```python
from build123d import *
from build123d import SkipClean  # not in build123d's __all__

# Parameters (mm, degrees)
F1_DEPTH = 10
F2_R     = 15
F3_DEPTH = 32
F4_DEPTH = 25
F5_DEPTH = 20


with BuildPart() as f1:
    # F0 (on Top) → F1 (new body)
    with BuildSketch(Plane.XY):
        with BuildLine():
            Line((-19.7133726581, 60.8366520235), (-69.7133726581, 60.8366520235))
            ThreePointArc((-69.7133726581, 60.8366520235), (-63.0146428473, 35.8366520235), (-69.7133726581, 10.8366520235))
            Line((-69.7133726581, 10.8366520235), (-19.7133726581, 10.8366520235))
            Line((-19.7133726581, 10.8366520235), (-19.7133726581, 60.8366520235))
        make_face()
    extrude(amount=F1_DEPTH)

    # F2 (on face) → F3 (join)
    with BuildSketch(Plane.XY.offset(10)):
        with Locations((-38.7318296711, 37.7283993232)):
            Circle(F2_R)
        with BuildLine():
            ThreePointArc((-35.6207755692, 50.8650405369), (-28.1429385494, 46.1024894119), (-25.2318296711, 37.7283993232))
            ThreePointArc((-25.2318296711, 37.7283993232), (-28.1429385494, 29.3543092346), (-35.6207755692, 24.5917581096))
            ThreePointArc((-35.6207755692, 24.5917581096), (-38.7318296711, 24.2283993232), (-41.8428837729, 24.5917581096))
            ThreePointArc((-41.8428837729, 24.5917581096), (-52.2318296711, 37.7283993232), (-41.8428837729, 50.8650405369))
            ThreePointArc((-41.8428837729, 50.8650405369), (-38.7318296711, 51.2283993232), (-35.6207755692, 50.8650405369))
        make_face(mode=Mode.SUBTRACT)
    extrude(amount=F3_DEPTH)

    # F2 (on face) → F4 (cut)
    with BuildSketch(Plane.XY.offset(10)):
        with BuildLine():
            Line((-41.8428837729, 24.5917581096), (-41.8428837729, 50.8650405369))
            ThreePointArc((-41.8428837729, 50.8650405369), (-52.2318296711, 37.7283993232), (-41.8428837729, 24.5917581096))
        make_face()
        with BuildLine():
            ThreePointArc((-35.6207755692, 24.5917581096), (-28.1429385494, 29.3543092346), (-25.2318296711, 37.7283993232))
            ThreePointArc((-25.2318296711, 37.7283993232), (-28.1429385494, 46.1024894119), (-35.6207755692, 50.8650405369))
            Line((-35.6207755692, 50.8650405369), (-35.6207755692, 24.5917581096))
        make_face()
    with SkipClean():  # cleaning this boolean's faces spoils the solid; the shape is the same uncleaned
        extrude(amount=-F4_DEPTH, mode=Mode.SUBTRACT)

    # F5 (add): a face of the model
    f5_faces = [f1.faces().sort_by_distance(p)[0] for p in [
        (-38.7318296711, 37.7283993232, 10),
    ]]
    with SkipClean():  # cleaning this boolean's faces spoils the solid; the shape is the same uncleaned
        extrude(f5_faces, amount=F5_DEPTH)


solid = f1.part
```
The listing builds one solid part. Answer for the finished solid, in the listing's coordinates (mm). A direction names the side the tool comes from. Round coordinates to 2 decimals unless told otherwise and drop trailing zeros. Write each loop counter-clockwise with the first axis right and the second up, starting at its lowest first coordinate (ties: lowest second). Pieces come first, ordered by that corner, then holes. Notation, with made-up numbers: (-7, 77) -> (51, 77) arc R21 cw to (51, 116) -> close; hole circle Ø8 at (62, 13). An arc over 180 degrees is marked (long way). Use CSV: the item, a comma, the result in double quotes. Start each with the question number.
(1) Section A-A on z = 6 is taken. Give the vertices of the cut face in (x, y), then the cut area to 3 significant figures.
(2) Section D-D on x = -45 is taken. Give the vertices of the cut face in (y, z).
(3) Section B-B on y = 37 is taken. Give the vertices of the cut face in (x, z), then the cut area to 3 significant figures.
(4) The mould has two halves that part along Y. Classify faces 3 (the face through (-44, 60.837, 5)), 4 (the face through (-19.713, 35, 5)), 5 (the face through (-63.016, 36.203, 4.93)), 6 (the face through (-35.621, 38, 15)): released by +Y, released by -Y, zero draft, split by the parting line, or undercut.
(5) Consider L1, parallel to X at y = 37.5, z = 32.5; L2, parallel to X at y = 35.5, z = 24.5; L3, parallel to X at y = 25.5, z = 11.5. Determine where each line is inside the solid, lowest interval first. Write a range as from..to.
(6) Each of these flat-tipped pins is pushed along its axis until it touches: pin 1 (10 mm diameter, centred on x = -32.5, z = 18.5, fed in from +Y); pin 2 (6 mm diameter, centred on y = 46, z = 21, fed in from -X) (3 decimals); pin 3 (3 mm diameter, centred on x = -40, y = 37, fed in from +Z); pin 4 (5 mm diameter, centred on x = -47.5, y = 37.5, fed in from -Z). Where does it stop, or does it pass through?
(7) Section C-C on z = 32.5 is taken. Give the vertices of the cut face in (x, y).
(8) Which of the six approach directions +Z, -Z, +X, -X, +Y, -Y give full straight-line access (tool end or side, diameter ignored) to faces 1 (the face through (-45, 10.837, 5)), 2 (the face through (-39, 38, 30))?
A:
1,outline,"(-69.71, 10.84) -> (-19.71, 10.84) -> (-19.71, 60.84) -> (-69.71, 60.84) arc R50 cw to start; hole (-41.84, 24.59) -> (-41.84, 50.87) arc R13.5 ccw to start; hole (-35.62, 24.59) arc R13.5 ccw to (-35.62, 50.87) -> close"
1,area,"1,870 mm²"
2,outline,"(10.84, 0) -> (25.77, 0) -> (25.77, 42) -> (24.1, 42) -> (24.1, 10) -> (10.84, 10) -> close; (49.68, 0) -> (60.84, 0) -> (60.84, 10) -> (51.36, 10) -> (51.36, 42) -> (49.68, 42) -> close"
3,outline,"(-63.03, 0) -> (-52.21, 0) -> (-52.21, 42) -> (-53.71, 42) -> (-53.71, 10) -> (-63.03, 10) -> close; (-41.84, 0) -> (-35.62, 0) -> (-35.62, 30) -> (-41.84, 30) -> close; (-25.25, 0) -> (-19.71, 0) -> (-19.71, 10) -> (-23.75, 10) -> (-23.75, 42) -> (-25.25, 42) -> close"
3,area,"446 mm²"
4,face 3,"released by +Y"
4,face 4,"zero draft"
4,face 5,"undercut"
4,face 6,"undercut"
5,L1,"x = -53.73..-52.23, -25.23..-23.73"
5,L2,"x = -53.57..-52.05, -41.84..-35.62, -25.42..-23.9"
5,L3,"x = -47.42..-44.45, -41.84..-35.62, -33.01..-30.04"
6,pin 1,"stops at y = 52.68"
6,pin 2,"stops at x = -52.775"
6,pin 3,"stops at z = 30"
6,pin 4,"passes through"
7,outline,"circle Ø30 at (-38.73, 37.73); hole circle Ø27 at (-38.73, 37.73)"
8,face 1,"+Z, -Z, +X, -X, -Y"
8,face 2,"+Z"
